Design review of the part built by this model. Coordinates are the model's own, in mm. A direction names the side the tool comes from. Coordinates: 2 decimals unless noted, no trailing zeros. Loops run counter-clockwise (first coordinate to the right, second up) from the corner with the lowest first, then second, coordinate; pieces in that order, holes last. Notation, with made-up numbers: (-34, -16) - (24, -16) arc R25 cw to (24, 22) - close; hole circle Ø8 at (-5.5, 44). An arc over 180 degrees is marked (long way). Return JSON: item names as keys, results as strings. Group by question number.
from build123d import *

# Parameters (mm, degrees)
SKETCH1_W           = 80
SKETCH1_H           = 30
BOSS_EXTRUDE2_DEPTH = 20
SKETCH4_W           = 20
SKETCH4_H           = 30
BOSS_EXTRUDE3_DEPTH = 50
SKETCH6_R           = 5
CUT_EXTRUDE2_DEPTH  = 50
SKETCH7_R           = 5
CUT_EXTRUDE4_DEPTH  = 50


with BuildPart() as part:
    # Sketch1 → Boss-Extrude2 (new body)
    with BuildSketch(Plane(origin=(0, 0, 0), x_dir=(1, 0, 0), z_dir=(0, 1, 0))):
        with Locations((40, 15)):
            Rectangle(SKETCH1_W, SKETCH1_H)
    extrude(amount=BOSS_EXTRUDE2_DEPTH)

    # Sketch4 → Boss-Extrude3 (add)
    with BuildSketch(Plane(origin=(0, 20, 0), x_dir=(1, 0, 0), z_dir=(0, 1, 0))):
        with Locations((10, 15)):
            Rectangle(SKETCH4_W, SKETCH4_H)
    extrude(amount=BOSS_EXTRUDE3_DEPTH)

    # Sketch6 → Cut-Extrude2 (cut)
    with BuildSketch(Plane(origin=(0, 20, 0), x_dir=(1, 0, 0), z_dir=(0, 1, 0))):
        with Locations(Location((60.018182297, 14.993207378, 0), (0, 0, 270))):
            Circle(SKETCH6_R)
    extrude(amount=-CUT_EXTRUDE2_DEPTH, mode=Mode.SUBTRACT)

    # Sketch7 → Cut-Extrude4 (cut)
    with BuildSketch(Plane(origin=(20, 0, 0), x_dir=(0, 0, -1), z_dir=(1, 0, 0))):
        with Locations((15, 50)):
            Circle(SKETCH7_R)
    extrude(amount=-CUT_EXTRUDE4_DEPTH, mode=Mode.SUBTRACT)


solid = part.part
Item 1: To check wall thickness, follow line 1 (Y direction, x = 7, z = -15); line 2 (Y direction, x = 28.5, z = -23.25). State the ranges of each line that lie inside material, in increasing order. Write a range as from..to.
Item 2: For P1, Ø9, axis at x = 50, z = -18.5, coming from the +Y side; P2, Ø8, axis at x = 18.5, z = -22.5, coming from the -Y side; P3, Ø4, axis at y = 57, z = -12.5, coming from the +X side, all flat-tipped, find the tip position at first contact; note any pin that passes through.
Item 3: Add section A-A (y = 50). State the section outline as (x, z) points, then the cut area to 3 significant figures.
Item 4: Draft analysis for pull direction Z (two halves, no side actions). For faces 3 (the face through (0, 35, -15)), 4 (the face through (31, 19, -30)), 5 (the face through (56.976, 10.14, -18.961)), state which applies: pulls with the +Z half, pulls with the -Z half, needs draft (parallel to the pull), parting line crosses it, or undercut.
Item 5: Add section D-D (z = -27.75). State the section outline as (x, y) points, then the cut area to 3 significant figures.
Item 6: Add section C-C (x = 61.5). State the section outline as (y, z) points.
Item 7: Add section B-B (z = -15). State the section outline as (x, y) points, then the cut area to 3 significant figures.
Item 8: For faces 1 (the face through (39, 0, -15)), 2 (the face through (50, 20, -15)), list the 3-axis set-ups (+Z, -Z, +X, -X, +Y, -Y) from which the entire face can be reached by the end or side of a thin tool; tool diameter is ignored.
Answers below:
{
 "1": {"line 1": "y = 0..45, 55..70", "line 2": "y = 0..20"},
 "2": {"P1": "stops at y = 20", "P2": "stops at y = 0", "P3": "stops at x = 20"},
 "3": {"outline": "(0, -30) - (20, -30) - (20, -20) - (0, -20) - close; (0, -10) - (20, -10) - (20, 0) - (0, 0) - close", "area": "400 mm^2"},
 "4": {"face 3": "needs draft", "face 4": "pulls with the -Z half", "face 5": "undercut"},
 "5": {"outline": "(0, 0) - (80, 0) - (80, 20) - (20, 20) - (20, 70) - (0, 70) - close", "area": "2,600 mm^2"},
 "6": {"outline": "(0, -30) - (20, -30) - (20, -19.77) - (0, -19.77) - close; (0, -10.22) - (20, -10.22) - (20, 0) - (0, 0) - close"},
 "7": {"outline": "(0, 0) - (55.02, 0) - (55.02, 20) - (20, 20) - (20, 45) - (0, 45) - close; (0, 55) - (20, 55) - (20, 70) - (0, 70) - close; (65.02, 0) - (80, 0) - (80, 20) - (65.02, 20) - close", "area": "2,200 mm^2"},
 "8": {"face 1": "+Z, -Z, +X, -X, -Y", "face 2": "+Z, -Z, +X, +Y"}
}
